from build123d import *

# Parameters (mm, degrees)
F0_W      = 5
F0_H      = 10
F0_H_2    = 5
F0_W_2    = 80
F0_H_3    = 35
F1_DEPTH  = 4
F3_D      = 3
F4_W      = 10
F4_H      = 10
F5_DEPTH  = 25
F7_D      = 10.5
F7_DEPTH  = 10.001
F9_D      = 10.5
F10_R     = 9.99999
F11_R     = 4.99999
F13_D     = 3.2
F13_DEPTH = 25
F13_TIP   = 0.9613769904
F14_R     = 1.5


# Not quite as in the source:
# - a fillet or chamfer is up to 0.001 mm smaller than in the source, because OpenCascade refuses the exact size
# - a feature names something its author has since deleted; it is built from what else it names


with BuildPart() as f1:
    # F0 (on Front) → F1 (new body)
    with BuildSketch(Plane.XZ):
        with Locations((-82.5, 50)):
            Rectangle(F0_W, F0_H)
        with Locations((-87.5, 50)):
            Rectangle(F0_W, F0_H)
        with Locations((-87.5, 5)):
            Rectangle(F0_W, F0_H)
        with Locations((-82.5, 5)):
            Rectangle(F0_W, F0_H)
        with Locations((2.5, 50)):
            Rectangle(F0_W, F0_H)
        with Locations((7.5, 50)):
            Rectangle(F0_W, F0_H)
        with Locations((2.5, 7.5)):
            Rectangle(F0_W, F0_H_2)
        with Locations((7.5, 7.5)):
            Rectangle(F0_W, F0_H_2)
        with Locations((7.5, 2.5)):
            Rectangle(F0_W, F0_H_2)
        with Locations((2.5, 2.5)):
            Rectangle(F0_W, F0_H_2)
        with Locations((-40, 50)):
            Rectangle(F0_W_2, F0_H)
        with Locations((2.5, 27.5)):
            Rectangle(F0_W, F0_H_3)
        with Locations((7.5, 27.5)):
            Rectangle(F0_W, F0_H_3)
        with Locations((-82.5, 27.5)):
            Rectangle(F0_W, F0_H_3)
        with Locations((-87.5, 27.5)):
            Rectangle(F0_W, F0_H_3)
    extrude(amount=-F1_DEPTH)

    # F3 (through all)
    with Locations(Plane.XZ):
        with Locations((5, 50), (-85, 50), (5, 5), (-85, 5)):
            Hole(F3_D / 2)

    # F4 (on Front) → F5 (join)
    with BuildSketch(Plane.XZ):
        with Locations((5, 22.5)):
            Rectangle(F4_W, F4_H)
        with Locations((5, 32.5)):
            Rectangle(F4_W, F4_H)
        with Locations((-85, 22.5)):
            Rectangle(F4_W, F4_H)
        with Locations((-85, 32.5)):
            Rectangle(F4_W, F4_H)
    extrude(amount=-F5_DEPTH)

    # F7 (through all, one way)
    with BuildSketch(Plane(origin=(0, 0, 0), x_dir=(0, 1, 0), z_dir=(-1, 0, 0))):
        with Locations((15, -27.5)):
            Circle(F7_D / 2)
    extrude(amount=-F7_DEPTH, mode=Mode.SUBTRACT)

    # F9 (through all)
    with Locations(Plane.YZ):
        with Locations((15, 27.5)):
            Hole(F9_D / 2)

    # F10 (radius 10 in the source; OpenCascade refuses exactly that, so slightly less here)
    f10_edges = [f1.edges().sort_by_distance(p)[0] for p in [
        (5, 25, 37.5),
        (5, 25, 17.5),
        (-85, 25, 37.5),
        (-85, 25, 17.5),
    ]]
    fillet(f10_edges, radius=F10_R)

    # F11 (radius 5 in the source; OpenCascade refuses exactly that, so slightly less here)
    f11_edges = [f1.edges().sort_by_distance(p)[0] for p in [
        (10, 2, 0),
        (-90, 2, 0),
        (-80, 2, 0),
        (-90, 2, 55),
        (10, 2, 55),
        (0, 2, 0),
    ]]
    fillet(f11_edges, radius=F11_R)

    # F13
    with Locations(Plane.XZ):
        with Locations((5, 27.5), (-85, 27.5)):
            Hole(F13_D / 2, depth=F13_DEPTH)
            with Locations((0, 0, -(F13_DEPTH + F13_TIP / 2))):  # 118° drill point
                Cone(0, F13_D / 2, F13_TIP, mode=Mode.SUBTRACT)

    # F14
    f14_edges = [f1.edges().sort_by_distance(p)[0] for p in [
        (-40, 4, 55),
        (10, 22.071071, 34.571071),
        (10, 4, 11.249995),
        (0, 22.071071, 34.571071),
        (0, 4, 41.25),
        (-40, 4, 45),
        (-80, 4, 41.25),
        (-80, 22.071071, 34.571071),
        (-90, 22.071071, 34.571071),
        (-90, 4, 11.249995),
    ]]
    fillet(f14_edges, radius=F14_R)


solid = f1.part
Work out the finished part from the listing and answer in its coordinate system (mm). A direction names the side the tool comes from. Give positions to 0.01 mm unless a question says otherwise; leave off trailing zeros. Order: outer loops, then holes, each group sorted by start corner. A loop starts at its lowest first (then second) coordinate and runs counter-clockwise, first axis right, second up. Notation, with made-up numbers: (46.25, 60.5) -> (79.25, 60.5) arc R29 ccw to (79.25, 97.5) -> close; hole circle Ø6 at (62.5, 71). An arc over 180 degrees is marked (long way). One line per item, written item: value.
Item 1: Determine the mould class of faces 1 (the flat face through (0, 9, 25)), 2 (the cylindrical face through (4.93, 19.85, 29.51)), 3 (the flat face through (5, 4, 10)), 4 (the cylindrical face through (-85.07, 10.15, 25.49)) for opening direction Y: released by +Y, released by -Y, zero draft, split by the parting line, or undercut.
Answer sheet:
face 1: zero draft
face 2: undercut
face 3: released by +Y
face 4: undercut
Item 2: Find section D-D, the plane x = -23. Give the vertices of the cut face in (y, z).
Answer sheet:
outline: (0, 45) -> (2.5, 45) arc R1.5 ccw to (4, 46.5) -> (4, 53.5) arc R1.5 ccw to (2.5, 55) -> (0, 55) -> close
Item 3: Find section A-A, the plane y = 8.25. Give the vertices of the cut face in (x, z).
Answer sheet:
outline: (-90, 19) arc R1.5 ccw to (-88.5, 17.5) -> (-81.5, 17.5) arc R1.5 ccw to (-80, 19) -> (-80, 36) arc R1.5 ccw to (-81.5, 37.5) -> (-88.5, 37.5) arc R1.5 ccw to (-90, 36) -> close; (0, 19) arc R1.5 ccw to (1.5, 17.5) -> (8.5, 17.5) arc R1.5 ccw to (10, 19) -> (10, 36) arc R1.5 ccw to (8.5, 37.5) -> (1.5, 37.5) arc R1.5 ccw to (0, 36) -> close; hole circle Ø3.2 at (-85, 27.5); hole circle Ø3.2 at (5, 27.5)
Item 4: Flat-ended cylindrical pins translate along their axes: P1, Ø17.5, axis at x = -50, z = 47, coming from the +Y side; P2, Ø4, axis at x = -1.5, y = 18.5, coming from the -Z side; P3, Ø5.5, axis at x = -84, y = 9, coming from the +Z side. Find the tip coordinate at first contact, or state that the pin passes through.
Answer sheet:
P1: y = 4
P2: z = 18.42
P3: z = 37.5
Item 5: A tool of negligible diameter and unlimited length cuts with its end or side. For faces 5 (the flat face through (5, 9, 17.5)), 6 (the flat face through (5, 9, 37.5)), 7 (the cylindrical face through (-83.4, 5.07, 27.57)), 8 (the cylindrical face through (-81, 1, 2)), from which of +Z, -Z, +X, -X, +Y, -Y can it reach the whole face along a straight path? Write none if from no direction.
Answer sheet:
face 5: -Z, +X, -X, +Y
face 6: +Z, +X, -X, +Y
face 7: +Y, -Y
face 8: -Z, +Y, -Y
Item 6: Straight lines are drawn through the part: probe 1 along Z at (x, y) = (-85, 1.4); probe 2 along X at (y, z) = (22.95, 27.5); probe 3 along X at (y, z) = (3.75, 24). For each, find the intervals that lie inside material, in ascending order.
Answer sheet:
probe 1: 0 to 3.5, 6.5 to 25.9, 29.1 to 48.5, 51.5 to 55
probe 2: -90 to -86.6, -83.4 to -80, 0 to 3.4, 6.6 to 10
probe 3: -90 to -80, 0 to 10
Item 7: Find section B-B, the plane z = 44. Give the vertices of the cut face in (x, y).
Answer sheet:
outline: (-90, 0) -> (-80, 0) -> (-80, 2.5) arc R1.5 ccw to (-81.5, 4) -> (-88.5, 4) arc R1.5 ccw to (-90, 2.5) -> close; (0, 0) -> (10, 0) -> (10, 2.5) arc R1.5 ccw to (8.5, 4) -> (1.5, 4) arc R1.5 ccw to (0, 2.5) -> close
Item 8: Find section C-C, the plane y = 12.5. Give the vertices of the cut face in (x, z).
Answer sheet:
outline: (-90, 19) arc R1.5 ccw to (-88.5, 17.5) -> (-81.5, 17.5) arc R1.5 ccw to (-80, 19) -> (-80, 22.88) -> (-90, 22.88) -> close; (-90, 32.12) -> (-80, 32.12) -> (-80, 36) arc R1.5 ccw to (-81.5, 37.5) -> (-88.5, 37.5) arc R1.5 ccw to (-90, 36) -> close; (0, 19) arc R1.5 ccw to (1.5, 17.5) -> (8.5, 17.5) arc R1.5 ccw to (10, 19) -> (10, 22.88) -> (0, 22.88) -> close; (0, 32.12) -> (10, 32.12) -> (10, 36) arc R1.5 ccw to (8.5, 37.5) -> (1.5, 37.5) arc R1.5 ccw to (0, 36) -> close
